from build123d import *


with BuildPart() as part:
    # Sketch1 → Revolve1 (revolve)
    with BuildSketch(Plane.XY, mode=Mode.PRIVATE) as revolve1_sk:
        Polygon((0, 0), (171, 0), (171, 5.5), (171, 6), (170.5, 6), (170.5, 5.5), (170, 5.5), (170, 6), (169.5, 6), (169.5, 5.5), (169, 5.5), (169, 6), (168.5, 6), (168.5, 5.5), (168, 5.5), (168, 6), (167.5, 6), (167.5, 5.5), (167, 5.5), (167, 6), (166.5, 6), (166.5, 5.5), (166, 5.5), (166, 6), (165.5, 6), (165.5, 5.5), (165, 5.5), (165, 6), (164.5, 6), (164.5, 5.5), (164, 5.5), (164, 6), (163.5, 6), (163.5, 5.5), (163, 5.5), (163, 6), (162.5, 6), (162.5, 5.5), (162, 5.5), (162, 6), (161.5, 6), (161.5, 5.5), (161, 5.5), (161, 6), (160.5, 6), (160.5, 5.5), (160, 5.5), (160, 6), (159.5, 6), (159.5, 5.5), (159, 5.5), (159, 6), (158.5, 6), (158.5, 5.5), (158, 5.5), (158, 6), (157.5, 6), (157.5, 5.5), (157, 5.5), (157, 6), (156.5, 6), (156.5, 5.5), (156, 5.5), (156, 6), (155.5, 6), (155.5, 5.5), (155, 5.5), (155, 6), (154.5, 6), (154.5, 5.5), (154, 5.5), (154, 6), (153.5, 6), (153.5, 5.5), (153, 5.5), (153, 6), (152.5, 6), (152.5, 5.5), (152, 5.5), (152, 6), (151.5, 6), (151.5, 5.5), (151, 5.5), (151, 6), (121, 6), (47, 6), (2, 6), (2, 5.5), (1, 5.5), (1, 6), (0, 6), align=None)
    revolve(revolve1_sk.sketch.rotate(Axis((0, 0, 0), (1, 0, 0)), 90), axis=Axis((0, 0, 0), (1, 0, 0)))


solid = part.part
Design review of the part built by this model. Coordinates are the model's own, in mm. A direction names the side the tool comes from. Coordinates: 2 decimals unless noted, no trailing zeros. Write each loop counter-clockwise with the first axis right and the second up, starting at its lowest first coordinate (ties: lowest second). Pieces come first, ordered by that corner, then holes. Notation, with made-up numbers: (-4.5, 59) - (30.5, 59) arc R16 ccw to (30.5, 76) - close; hole circle Ø4 at (10, 80). An arc over 180 degrees is marked (long way). One line per item, written item: value.
1) Insertion check: pin 1 (3 mm diameter, centred on x = 50, y = 4, fed in from -Z); pin 2 (1.5 mm diameter, centred on x = 130, y = 2.5, fed in from -Z); pin 3 (1 mm diameter, centred on x = 102.5, z = 3.5, fed in from +Y). Each pin has a flat end and moves straight along its axis. Give the tip position at first contact, or say it passes through.
Answer sheet:
pin 1: stops at z = -5.45
pin 2: stops at z = -5.74
pin 3: stops at y = 5.2
2) Add section A-A (x = 140). State the section outline as (y, z) points, plus the area to 3 significant figures.
Answer sheet:
outline: circle Ø12 at (0, 0)
area: 113 mm2
3) For faces 3 (the face through (162.746, -1.802, 5.723)), 4 (the face through (158, 5, -3)), list the 3-axis set-ups (+Z, -Z, +X, -X, +Y, -Y) from which the entire face can be reached by the end or side of a thin tool; tool diameter is ignored.
Answer sheet:
face 3: +X, -X
face 4: none
4) Mouldability with a two-part tool opening along X and no side actions: class faces 1 (the face through (165.746, -1.802, 5.723)), 2 (the face through (165.5, 5, 3)) as +X half, -X half, draft (parallel to the pull), parting line (faces both ways), or undercut.
Answer sheet:
face 1: draft
face 2: undercut
5) To check wall thickness, follow probe 1 along Y at (x, z) = (144, -0.25); probe 2 along Z at (x, y) = (129, -0.5); probe 3 along Z at (x, y) = (62, 2.5). State the ranges of each line that lie inside material, in increasing order.
Answer sheet:
probe 1: y = -5.99 to 5.99
probe 2: z = -5.98 to 5.98
probe 3: z = -5.45 to 5.45
